Verification items for the finished model (mm, model axes). A direction names the side the tool comes from. Give positions to 0.01 mm unless a question says otherwise; leave off trailing zeros. Order: outer loops, then holes, each group sorted by start corner. A loop starts at its lowest first (then second) coordinate and runs counter-clockwise, first axis right, second up. Notation, with made-up numbers: (48, 6) - (69, 6) arc R13 cw to (69, 21) - close; hole circle Ø6 at (76.5, 2.5). An arc over 180 degrees is marked (long way). Answer as a JSON object with one key per item and string values. Group by question number.
(1) Thickness scan on line 1 (X direction, y = -9, z = 0); line 2 (Y direction, x = -7.25, z = -9.25); line 3 (Z direction, x = 9, y = 4.75). Record the ranges inside material, lowest first.
(2) Depth check by flat-ended pin: pin 1 Ø3 at (y, z) = (10, 8.5) entering from -X; pin 2 Ø4 at (x, y) = (-5.5, 7.5) entering from -Z; pin 3 Ø6 at (y, z) = (7, 8) entering from -X. Enter the tip coordinate at first touch or a pass-through.
(3) Section check A-A (x = 0). Record the boundary of the cut face in (y, z).
(4) Access from +Z, -Z, +X, -X, +Y, -Y to the whole of each face (thin tool, end or side, straight path). Record for faces 5 (the face through (-7.81, 13.94, -1.73)), 6 (the face through (-8.036, -0.112, 3.54)), 7 (the face through (7.643, -0.112, 7.752)).
(5) Mould release check, pull along Z, two halves, no side actions. Record for faces 1 (the face through (7.084, -0.112, 5.189)), 2 (the face through (-8.51, -0.11, 6.79)), 3 (the face through (8.596, 0.112, -1.792)), 4 (the face through (-8.5, 0.11, -6.79)): +Z half, -Z half, draft (parallel to the pull), parting line (faces both ways), or undercut.
(6) Section check C-C (x = -3.2). Record the boundary of the cut face in (y, z), then the cut area to 3 significant figures.
(7) Section check B-B (y = 13). Record the boundary of the cut face in (x, z).
```python
from build123d import *

# Parameters (mm, degrees)
SKETCH1_R           = 4
BOSS_EXTRUDE1_DEPTH = 8
SKETCH2_R           = 8
SKETCH2_R_2         = 4
BOSS_EXTRUDE2_DEPTH = 10
SKETCH2_3_R         = 14
SKETCH2_3_R_2       = 8
SKETCH2_3_R_3       = 4
BOSS_EXTRUDE3_DEPTH = 2


with BuildPart() as part:
    # Sketch1 → Boss-Extrude1 (new, symmetric)
    with BuildSketch(Plane(origin=(0, 0, 0), x_dir=(1, 0, 0), z_dir=(0, 1, 0))):
        with BuildLine():
            ThreePointArc((10.430731661, 0.607363835), (8.588743102, 1.825593703), (9.775984656, 3.687706308))
            ThreePointArc((9.775984656, 3.687706308), (10.132691352, 3.967450083), (10.145367447, 4.420589756))
            ThreePointArc((10.145367447, 4.420589756), (10.127694476, 4.460930288), (10.109861101, 4.501200167))
            ThreePointArc((10.109861101, 4.501200167), (10.091867606, 4.541398755), (10.073714274, 4.581525417))
            ThreePointArc((10.073714274, 4.581525417), (9.728483908, 4.875314866), (9.281910401, 4.797415253))
            ThreePointArc((9.281910401, 4.797415253), (7.103671393, 5.161119372), (7.430881092, 7.345138528))
            ThreePointArc((7.430881092, 7.345138528), (7.64296683, 7.745782868), (7.470238509, 8.16490239))
            ThreePointArc((7.470238509, 8.16490239), (7.437685474, 8.194567054), (7.405014641, 8.224101932))
            ThreePointArc((7.405014641, 8.224101932), (7.372226526, 8.253506556), (7.339321649, 8.282780461))
            ThreePointArc((7.339321649, 8.282780461), (6.904443081, 8.410752637), (6.52816251, 8.157949991))
            ThreePointArc((6.52816251, 8.157949991), (4.390310366, 7.604240615), (3.80091068, 9.732529569))
            ThreePointArc((3.80091068, 9.732529569), (3.831703908, 10.184799426), (3.503437469, 10.497429225))
            ThreePointArc((3.503437469, 10.497429225), (3.461633085, 10.511288732), (3.419773876, 10.52498176))
            ThreePointArc((3.419773876, 10.52498176), (3.377860505, 10.538508093), (3.335893634, 10.551867516))
            ThreePointArc((3.335893634, 10.551867516), (2.886561321, 10.491894868), (2.645636014, 10.107901062))
            ThreePointArc((2.645636014, 10.107901062), (0.917824792, 8.732519573), (-0.486271719, 10.43707783))
            ThreePointArc((-0.486271719, 10.43707783), (-0.642095428, 10.862771638), (-1.069139738, 11.01485518))
            ThreePointArc((-1.069139738, 11.01485518), (-1.112967112, 11.010513096), (-1.156776859, 11.005996626))
            ThreePointArc((-1.156776859, 11.005996626), (-1.200568284, 11.001305842), (-1.244340695, 10.996440818))
            ThreePointArc((-1.244340695, 10.996440818), (-1.630433115, 10.758893161), (-1.694344984, 10.310104213))
            ThreePointArc((-1.694344984, 10.310104213), (-2.713361027, 8.350866564), (-4.68937332, 9.336960516))
            ThreePointArc((-4.68937332, 9.336960516), (-5.004870632, 9.662471948), (-5.456852971, 9.627712608))
            ThreePointArc((-5.456852971, 9.627712608), (-5.495125185, 9.605919718), (-5.533310366, 9.583974688))
            ThreePointArc((-5.533310366, 9.583974688), (-5.57140791, 9.561877866), (-5.609417214, 9.539629602))
            ThreePointArc((-5.609417214, 9.539629602), (-5.865510854, 9.165581084), (-5.741358341, 8.729596681))
            ThreePointArc((-5.741358341, 8.729596681), (-5.875382075, 6.525272861), (-8.081639672, 6.622397905))
            ThreePointArc((-8.081639672, 6.622397905), (-8.502258236, 6.791443078), (-8.901026752, 6.575851062))
            ThreePointArc((-8.901026752, 6.575851062), (-8.927126192, 6.540375554), (-8.953084242, 6.504796459))
            ThreePointArc((-8.953084242, 6.504796459), (-8.978900494, 6.469114341), (-9.004574536, 6.433329764))
            ThreePointArc((-9.004574536, 6.433329764), (-9.086388479, 5.987456771), (-8.795638682, 5.639662576))
            ThreePointArc((-8.795638682, 5.639662576), (-8.021496185, 3.571400201), (-10.076517106, 2.762762534))
            ThreePointArc((-10.076517106, 2.762762534), (-10.52952815, 2.746112001), (-10.806132144, 2.386965126))
            ThreePointArc((-10.806132144, 2.386965126), (-10.815545979, 2.343941039), (-10.824788517, 2.300879828))
            ThreePointArc((-10.824788517, 2.300879828), (-10.833859611, 2.257782175), (-10.842759117, 2.214648764))
            ThreePointArc((-10.842759117, 2.214648764), (-10.73614699, 1.774046788), (-10.32907319, 1.574579578))
            ThreePointArc((-10.32907319, 1.574579578), (-8.780620732, 0), (-10.32907319, -1.574579578))
            ThreePointArc((-10.32907319, -1.574579578), (-10.73614699, -1.774046788), (-10.842759117, -2.214648764))
            ThreePointArc((-10.842759117, -2.214648764), (-10.833859611, -2.257782175), (-10.824788517, -2.300879828))
            ThreePointArc((-10.824788517, -2.300879828), (-10.815545979, -2.343941039), (-10.806132144, -2.386965126))
            ThreePointArc((-10.806132144, -2.386965126), (-10.52952815, -2.746112001), (-10.076517106, -2.762762534))
            ThreePointArc((-10.076517106, -2.762762534), (-8.021496185, -3.571400201), (-8.795638682, -5.639662576))
            ThreePointArc((-8.795638682, -5.639662576), (-9.086388479, -5.987456771), (-9.004574536, -6.433329764))
            ThreePointArc((-9.004574536, -6.433329764), (-8.978900494, -6.469114341), (-8.953084242, -6.504796459))
            ThreePointArc((-8.953084242, -6.504796459), (-8.927126192, -6.540375554), (-8.901026752, -6.575851062))
            ThreePointArc((-8.901026752, -6.575851062), (-8.502258236, -6.791443078), (-8.081639672, -6.622397905))
            ThreePointArc((-8.081639672, -6.622397905), (-5.875382075, -6.525272861), (-5.741358341, -8.729596681))
            ThreePointArc((-5.741358341, -8.729596681), (-5.865510854, -9.165581084), (-5.609417214, -9.539629602))
            ThreePointArc((-5.609417214, -9.539629602), (-5.57140791, -9.561877866), (-5.533310366, -9.583974688))
            ThreePointArc((-5.533310366, -9.583974688), (-5.495125185, -9.605919718), (-5.456852971, -9.627712608))
            ThreePointArc((-5.456852971, -9.627712608), (-5.004870632, -9.662471948), (-4.68937332, -9.336960516))
            ThreePointArc((-4.68937332, -9.336960516), (-2.713361027, -8.350866564), (-1.694344984, -10.310104213))
            ThreePointArc((-1.694344984, -10.310104213), (-1.630433115, -10.758893161), (-1.244340695, -10.996440818))
            ThreePointArc((-1.244340695, -10.996440818), (-1.200568284, -11.001305842), (-1.156776859, -11.005996626))
            ThreePointArc((-1.156776859, -11.005996626), (-1.112967112, -11.010513096), (-1.069139738, -11.01485518))
            ThreePointArc((-1.069139738, -11.01485518), (-0.642095428, -10.862771638), (-0.486271719, -10.43707783))
            ThreePointArc((-0.486271719, -10.43707783), (0.917824792, -8.732519573), (2.645636014, -10.107901062))
            ThreePointArc((2.645636014, -10.107901062), (2.886561321, -10.491894868), (3.335893634, -10.551867516))
            ThreePointArc((3.335893634, -10.551867516), (3.377860505, -10.538508093), (3.419773876, -10.52498176))
            ThreePointArc((3.419773876, -10.52498176), (3.461633085, -10.511288732), (3.503437469, -10.497429225))
            ThreePointArc((3.503437469, -10.497429225), (3.831703908, -10.184799426), (3.80091068, -9.732529569))
            ThreePointArc((3.80091068, -9.732529569), (4.390310366, -7.604240615), (6.52816251, -8.157949991))
            ThreePointArc((6.52816251, -8.157949991), (6.904443081, -8.410752637), (7.339321649, -8.282780461))
            ThreePointArc((7.339321649, -8.282780461), (7.372226526, -8.253506556), (7.405014641, -8.224101932))
            ThreePointArc((7.405014641, -8.224101932), (7.437685474, -8.194567054), (7.470238509, -8.16490239))
            ThreePointArc((7.470238509, -8.16490239), (7.64296683, -7.745782868), (7.430881092, -7.345138528))
            ThreePointArc((7.430881092, -7.345138528), (7.103671393, -5.161119372), (9.281910401, -4.797415253))
            ThreePointArc((9.281910401, -4.797415253), (9.728483908, -4.875314866), (10.073714274, -4.581525417))
            ThreePointArc((10.073714274, -4.581525417), (10.091867606, -4.541398755), (10.109861101, -4.501200167))
            ThreePointArc((10.109861101, -4.501200167), (10.127694476, -4.460930288), (10.145367447, -4.420589756))
            ThreePointArc((10.145367447, -4.420589756), (10.132691352, -3.967450083), (9.775984656, -3.687706308))
            ThreePointArc((9.775984656, -3.687706308), (8.588743102, -1.825593703), (10.430731661, -0.607363835))
            ThreePointArc((10.430731661, -0.607363835), (10.870381486, -0.496890864), (11.066270185, -0.088083006))
            ThreePointArc((11.066270185, -0.088083006), (11.066533095, -0.044041852), (11.066620732, 0))
            ThreePointArc((11.066620732, 0), (11.066533095, 0.044041852), (11.066270185, 0.088083006))
            ThreePointArc((11.066270185, 0.088083006), (10.870381486, 0.496890864), (10.430731661, 0.607363835))
        make_face()
        with Locations(Location((0, 0, 0), (0, 0, 270))):
            Circle(SKETCH1_R, mode=Mode.SUBTRACT)
    extrude(amount=BOSS_EXTRUDE1_DEPTH, both=True)

    # Sketch2 → Boss-Extrude2 (add)
    with BuildSketch(Plane(origin=(0, 8, 0), x_dir=(1, 0, 0), z_dir=(0, 1, 0))):
        with Locations(Location((0, 0, 0), (0, 0, 270))):
            Circle(SKETCH2_R)
        with Locations(Location((0, 0, 0), (0, 0, 270))):
            Circle(SKETCH2_R_2, mode=Mode.SUBTRACT)
    extrude(amount=BOSS_EXTRUDE2_DEPTH)

    # Sketch2_3 → Boss-Extrude3 (add)
    # profile 1 of 2: a face of its own
    with BuildSketch(Plane(origin=(0, 8, 0), x_dir=(1, 0, 0), z_dir=(0, 1, 0))):
        with Locations(Location((0, 0, 0), (0, 0, 270))):
            Circle(SKETCH2_3_R)
        with Locations(Location((0, 0, 0), (0, 0, 270))):
            Circle(SKETCH2_3_R_2, mode=Mode.SUBTRACT)
    # profile 2 of 2: a face of its own
    with BuildSketch(Plane(origin=(0, 8, 0), x_dir=(1, 0, 0), z_dir=(0, 1, 0))):
        with Locations(Location((0, 0, 0), (0, 0, 270))):
            Circle(SKETCH2_3_R_2)
        with Locations(Location((0, 0, 0), (0, 0, 270))):
            Circle(SKETCH2_3_R_3, mode=Mode.SUBTRACT)
    boss_extrude3 = extrude(amount=BOSS_EXTRUDE3_DEPTH)

    # Mirror1: Boss-Extrude3 across plane
    add(boss_extrude3.mirror(Plane.ZX))


solid = part.part
```
Solutions:
{
 "1": {"line 1": "x = -14 to -4, 4 to 14", "line 2": "y = -10 to -8, 8 to 10", "line 3": "z = -4.64 to -3.25, -1.06 to 1.06, 3.25 to 4.64"},
 "2": {"pin 1": "stops at x = -12.12", "pin 2": "stops at z = -13.54", "pin 3": "stops at x = -13.01"},
 "3": {"outline": "(-10, -14) - (-8, -14) - (-8, -9.15) - (8, -9.15) - (8, -14) - (10, -14) - (10, -8) - (18, -8) - (18, -4) - (-10, -4) - close; (-10, 4) - (18, 4) - (18, 8) - (10, 8) - (10, 14) - (8, 14) - (8, 9.15) - (-8, 9.15) - (-8, 14) - (-10, 14) - close"},
 "4": {"face 5": "+Y", "face 6": "none", "face 7": "+X"},
 "5": {"face 1": "undercut", "face 2": "+Z half", "face 3": "undercut", "face 4": "-Z half"},
 "6": {"outline": "(-10, -13.63) - (-8, -13.63) - (-8, -8.27) - (8, -8.27) - (8, -13.63) - (10, -13.63) - (10, -7.33) - (18, -7.33) - (18, -2.4) - (-10, -2.4) - close; (-10, 2.4) - (18, 2.4) - (18, 7.33) - (10, 7.33) - (10, 13.63) - (8, 13.63) - (8, 8.27) - (-8, 8.27) - (-8, 13.63) - (-10, 13.63) - close", "area": "357 mm2"},
 "7": {"outline": "circle Ø16 at (0, 0); hole circle Ø8 at (0, 0)"}
}
